Design review of the part built by this model. Coordinates are the model's own, in mm. A direction names the side the tool comes from. Round coordinates to 2 decimals unless told otherwise and drop trailing zeros. Order: outer loops, then holes, each group sorted by start corner. A loop starts at its lowest first (then second) coordinate and runs counter-clockwise, first axis right, second up. Notation, with made-up numbers: (17, -11) - (27, -11) arc R15 ccw to (27, 0) - close; hole circle Ø10 at (-1, 19). An arc over 180 degrees is marked (long way). Write item = value, one per line.
from build123d import *

# Parameters (mm, degrees)
SKETCH1_W           = 53
SKETCH1_H           = 53
BOSS_EXTRUDE1_DEPTH = 2
SKETCH2_W           = 36
SKETCH2_H           = 5
BOSS_EXTRUDE2_DEPTH = 5.9
SKETCH3_R           = 1.6
CUT_EXTRUDE1_DEPTH  = 3.6
CUT_EXTRUDE2_START  = 3.6
SKETCH4_R           = 1.6
CUT_EXTRUDE2_DEPTH  = 3.6
FILLET1_R           = 2.6


with BuildPart() as part:
    # Sketch1 → Boss-Extrude1 (new body)
    with BuildSketch(Plane(origin=(0, 0, 0), x_dir=(1, 0, 0), z_dir=(0, 1, 0))):
        Rectangle(SKETCH1_W, SKETCH1_H)
    extrude(amount=BOSS_EXTRUDE1_DEPTH)

    # Sketch2 → Boss-Extrude2 (add)
    with BuildSketch(Plane(origin=(0, 2, 0), x_dir=(1, 0, 0), z_dir=(0, 1, 0))):
        with Locations((0, 24)):
            Rectangle(SKETCH2_W, SKETCH2_H)
        with Locations((0, -24)):
            Rectangle(SKETCH2_W, SKETCH2_H)
    extrude(amount=BOSS_EXTRUDE2_DEPTH)

    # Sketch3 → Cut-Extrude1 (cut)
    with BuildSketch(Plane(origin=(18, 0, 0), x_dir=(0, 0, -1), z_dir=(1, 0, 0))):
        with Locations((-24, 4.8)):
            Circle(SKETCH3_R)
        with Locations(Location((24, 4.8, 0), (0, 0, 180))):
            Circle(SKETCH3_R)
    extrude(amount=-CUT_EXTRUDE1_DEPTH, mode=Mode.SUBTRACT)

    # Sketch4 → Cut-Extrude2 (cut)
    with BuildSketch(Plane(origin=(-18, 0, -18), x_dir=(0, 0, -1), z_dir=(1, 0, 0)).offset(CUT_EXTRUDE2_START)):
        with Locations((-42, 4.8)):
            Circle(SKETCH4_R)
        with Locations(Location((6, 4.8, 0), (0, 0, 180))):
            Circle(SKETCH4_R)
    extrude(amount=-CUT_EXTRUDE2_DEPTH, mode=Mode.SUBTRACT)

    # Fillet1
    # the kernel refuses this fillet: 2.6 mm, written as the material it takes off along each edge
    with BuildSketch(Plane(origin=(-24.5, 7.9, -26.5), x_dir=(0, -1, 0), z_dir=(1, 0, 0)), Plane(origin=(24.5, 7.9, -21.5), x_dir=(0, -1, 0), z_dir=(-1, 0, 0)), Plane(origin=(24.5, 7.9, 26.5), x_dir=(0, -1, 0), z_dir=(-1, 0, 0))) as fillet1_piece_1:
        with BuildLine():
            CenterArc((FILLET1_R, -FILLET1_R), FILLET1_R, 90, 90)
            Line((0, -FILLET1_R), (0, 0))
            Line((0, 0), (FILLET1_R, 0))
        make_face()
    extrude(amount=49, mode=Mode.SUBTRACT)
    with BuildSketch(Plane(origin=(-24.5, 7.9, 21.5), x_dir=(0, 0, 1), z_dir=(1, 0, 0))) as fillet1_piece_2:
        with BuildLine():
            CenterArc((FILLET1_R, FILLET1_R), FILLET1_R, 180, 90)
            Line((0, FILLET1_R), (0, 0))
            Line((0, 0), (FILLET1_R, 0))
        make_face()
    extrude(amount=49, mode=Mode.SUBTRACT)


solid = part.part
Item 1: Take a section at A-A, the plane x = -16. State the section outline as (y, z) points.
Data:
outline = (0, -26.5) - (5.3, -26.5) arc R2.6 ccw to (7.9, -24) arc R2.6 ccw to (5.3, -21.5) - (2, -21.5) - (2, 21.5) - (5.3, 21.5) arc R2.6 ccw to (7.9, 24) arc R2.6 ccw to (5.3, 26.5) - (0, 26.5) - close; hole circle Ø3.2 at (4.8, -24); hole circle Ø3.2 at (4.8, 24)
Item 2: Take a section at C-C, the plane x = -10.5. State the section outline as (y, z) points.
Data:
outline = (0, -26.5) - (5.3, -26.5) arc R2.6 ccw to (7.9, -24) arc R2.6 ccw to (5.3, -21.5) - (2, -21.5) - (2, 21.5) - (5.3, 21.5) arc R2.6 ccw to (7.9, 24) arc R2.6 ccw to (5.3, 26.5) - (0, 26.5) - close
Item 3: Insertion check: P1, Ø4, axis at y = 4.8, z = -24, coming from the +X side; P2, Ø3, axis at y = 4.8, z = 24, coming from the +X side; P3, Ø1.6, axis at y = 4, z = -23.5, coming from the -X side. Each pin has a flat end and moves straight along its axis. Give the tip position at first contact, or say it passes through.
Data:
P1 = 18
P2 = 14.4
P3 = -18
Item 4: The part is to be moulded in two halves that separate along Z. For faces 5 (the face through (0, 3, -26.5)), 6 (the face through (-18, 5, 22)), 7 (the face through (14.4, 5, 24)), say which applies: +Z half, -Z half, draft (parallel to the pull), parting line (faces both ways), or undercut.
Data:
face_5 = -Z half
face_6 = draft
face_7 = undercut
Item 5: For faces 1 (the face through (-0.252, 7.083, 22.207)), 2 (the face through (16.23, 3.24, 24.35)), 3 (the face through (-16.175, 3.214, -24.208)), 4 (the face through (18, 5, -26)), list the 3-axis set-ups (+Z, -Z, +X, -X, +Y, -Y) from which the entire face can be reached by the end or side of a thin tool; tool diameter is ignored.
Data:
face_1 = +X, -X, +Y
face_2 = +X
face_3 = -X
face_4 = +Z, -Z, +X, +Y
Item 6: Take a section at D-D, the plane z = 12.5. State the section outline as (x, y) points, and give its area (3 significant figures).
Data:
outline = (-26.5, 0) - (26.5, 0) - (26.5, 2) - (-26.5, 2) - close
area = 106 mm2
Item 7: For line 1 along Y through (x, z) = (15, -24); line 2 along Z through (x, y) = (-14.5, 3.5); line 3 along Z through (x, y) = (-14, 3.25), list the stretches that pass through material, from the lowest coordinate up. Write a range as [from, to].
Data:
line_1 = [0, 3.2], [6.4, 7.9]
line_2 = [-26.5, -24.93], [-23.07, -21.5], [21.5, 23.07], [24.93, 26.5]
line_3 = [-26.5, -21.5], [21.5, 26.5]
Item 8: Take a section at B-B, the plane y = 7.25. State the section outline as (x, z) points, and give its area (3 significant figures).
Data:
outline = (-18, -25.62) - (18, -25.62) - (18, -22.38) - (-18, -22.38) - close; (-18, 22.38) - (18, 22.38) - (18, 25.62) - (-18, 25.62) - close
area = 233 mm2
